For this review, take the finished solid that the model builds, in its own axes (mm). A direction names the side the tool comes from. Round coordinates to 2 decimals unless told otherwise and drop trailing zeros. Write each loop counter-clockwise with the first axis right and the second up, starting at its lowest first coordinate (ties: lowest second). Pieces come first, ordered by that corner, then holes. Notation, with made-up numbers: (43, 7.25) -> (102, 7.25) arc R34 ccw to (102, 46.25) -> close; hole circle Ø9 at (84, -10). An arc over 180 degrees is marked (long way). Write item = value, one per line. Start each with the question number.
```python
from build123d import *

# Parameters (mm, degrees)
SKETCH1_W           = 85.2
SKETCH1_H           = 85.2
BOSS_EXTRUDE1_DEPTH = 6.35
CUT_EXTRUDE1_REACH  = 62.579
SKETCH2_R           = 6.6675
CUT_EXTRUDE2_REACH  = 62.579
SKETCH3_R           = 2.6162
CUT_EXTRUDE3_REACH  = 62.579
SKETCH5_R           = 2.665
CIRPATTERN1_COUNT   = 4
CUT_EXTRUDE4_REACH  = 62.579
SKETCH6_W           = 85.2
SKETCH6_H           = 85.2
FILLET1_R           = 12.7


with BuildPart() as part:
    # Sketch1 → Boss-Extrude1 (new body)
    with BuildSketch(Plane(origin=(0, 0, 0), x_dir=(1, 0, 0), z_dir=(0, 1, 0))):
        Rectangle(SKETCH1_W, SKETCH1_H)
    extrude(amount=BOSS_EXTRUDE1_DEPTH)

    # Sketch2 → Cut-Extrude1 (cut, up to next)
    with BuildSketch(Plane(origin=(0, 6.35, 0), x_dir=(1, 0, 0), z_dir=(0, 1, 0)), mode=Mode.PRIVATE) as cut_extrude1_sk1:
        with Locations(Location((0, 0, 0), (0, 0, 270))):
            Circle(SKETCH2_R)
    cut_extrude1_tool1 = extrude(cut_extrude1_sk1.sketch, amount=-CUT_EXTRUDE1_REACH, mode=Mode.PRIVATE) & part.part
    add(cut_extrude1_tool1.solids().sort_by_distance((0, 6.35, 0))[0], mode=Mode.SUBTRACT)

    # Sketch3 → Cut-Extrude2 (cut, up to next)
    with BuildSketch(Plane(origin=(0, 6.35, 0), x_dir=(1, 0, 0), z_dir=(0, 1, 0)), mode=Mode.PRIVATE) as cut_extrude2_sk1:
        with Locations(Location((26.042742751, -26.042742751, 0), (0, 0, 270))):
            Circle(SKETCH3_R)
    cut_extrude2_tool1 = extrude(cut_extrude2_sk1.sketch, amount=-CUT_EXTRUDE2_REACH, mode=Mode.PRIVATE) & part.part
    # Sketch3 → Cut-Extrude2 (cut, up to next)
    with BuildSketch(Plane(origin=(0, 6.35, 0), x_dir=(1, 0, 0), z_dir=(0, 1, 0)), mode=Mode.PRIVATE) as cut_extrude2_sk2:
        with Locations(Location((-26.042742751, -26.042742751, 0), (0, 0, 270))):
            Circle(SKETCH3_R)
    cut_extrude2_tool2 = extrude(cut_extrude2_sk2.sketch, amount=-CUT_EXTRUDE2_REACH, mode=Mode.PRIVATE) & part.part
    # Sketch3 → Cut-Extrude2 (cut, up to next)
    with BuildSketch(Plane(origin=(0, 6.35, 0), x_dir=(1, 0, 0), z_dir=(0, 1, 0)), mode=Mode.PRIVATE) as cut_extrude2_sk3:
        with Locations(Location((26.042742751, 26.042742751, 0), (0, 0, 90))):
            Circle(SKETCH3_R)
    cut_extrude2_tool3 = extrude(cut_extrude2_sk3.sketch, amount=-CUT_EXTRUDE2_REACH, mode=Mode.PRIVATE) & part.part
    # Sketch3 → Cut-Extrude2 (cut, up to next)
    with BuildSketch(Plane(origin=(0, 6.35, 0), x_dir=(1, 0, 0), z_dir=(0, 1, 0)), mode=Mode.PRIVATE) as cut_extrude2_sk4:
        with Locations(Location((-26.042742751, 26.042742751, 0), (0, 0, 90))):
            Circle(SKETCH3_R)
    cut_extrude2_tool4 = extrude(cut_extrude2_sk4.sketch, amount=-CUT_EXTRUDE2_REACH, mode=Mode.PRIVATE) & part.part
    add(cut_extrude2_tool1.solids().sort_by_distance((26.042743, 6.35, 26.042743))[0], mode=Mode.SUBTRACT)
    add(cut_extrude2_tool2.solids().sort_by_distance((-26.042743, 6.35, 26.042743))[0], mode=Mode.SUBTRACT)
    add(cut_extrude2_tool3.solids().sort_by_distance((26.042743, 6.35, -26.042743))[0], mode=Mode.SUBTRACT)
    add(cut_extrude2_tool4.solids().sort_by_distance((-26.042743, 6.35, -26.042743))[0], mode=Mode.SUBTRACT)

    # Sketch5 → Cut-Extrude3 (cut, up to next)
    with BuildSketch(Plane(origin=(0, 6.35, 0), x_dir=(1, 0, 0), z_dir=(0, 1, 0)), mode=Mode.PRIVATE) as cut_extrude3_sk1:
        with Locations(Location((-34.75, -34.75, 0), (0, 0, 270))):
            Circle(SKETCH5_R)
    cut_extrude3_tool1 = extrude(cut_extrude3_sk1.sketch, amount=-CUT_EXTRUDE3_REACH, mode=Mode.PRIVATE) & part.part
    cut_extrude3 = cut_extrude3_tool1.solids().sort_by_distance((-34.75, 6.35, 34.75))[0]
    add(cut_extrude3, mode=Mode.SUBTRACT)

    # CirPattern1: Cut-Extrude3 ×4 about axis
    cirpattern1_axis = Axis((0, 0, 0), (0, 1, 0))
    for i in range(1, CIRPATTERN1_COUNT):
        add(cut_extrude3.rotate(cirpattern1_axis, i * 360 / CIRPATTERN1_COUNT), mode=Mode.SUBTRACT)

    # Sketch6 → Cut-Extrude4 (cut, up to next)
    with BuildSketch(Plane(origin=(0, 6.35, 0), x_dir=(1, 0, 0), z_dir=(0, 1, 0)), mode=Mode.PRIVATE) as cut_extrude4_sk1:
        Rectangle(SKETCH6_W, SKETCH6_H)
        with BuildLine():
            Line((31.75, -22.769743879), (39.240128061, -30.259871939))
            ThreePointArc((39.240128061, -30.259871939), (40.616635031, -32.319960204), (41.1, -34.75))
            ThreePointArc((41.1, -34.75), (37.180039796, -40.616635031), (30.259871939, -39.240128061))
            Line((30.259871939, -39.240128061), (22.769743879, -31.75))
            Line((22.769743879, -31.75), (-22.769743879, -31.75))
            Line((-22.769743879, -31.75), (-30.259871939, -39.240128061))
            ThreePointArc((-30.259871939, -39.240128061), (-39.240128061, -39.240128061), (-39.240128061, -30.259871939))
            Line((-39.240128061, -30.259871939), (-31.75, -22.769743879))
            Line((-31.75, -22.769743879), (-31.75, 22.769743879))
            Line((-31.75, 22.769743879), (-39.240128061, 30.259871939))
            ThreePointArc((-39.240128061, 30.259871939), (-39.240128061, 39.240128061), (-30.259871939, 39.240128061))
            Line((-30.259871939, 39.240128061), (-22.769743879, 31.75))
            Line((-22.769743879, 31.75), (22.769743879, 31.75))
            Line((22.769743879, 31.75), (30.259871939, 39.240128061))
            ThreePointArc((30.259871939, 39.240128061), (37.180039796, 40.616635031), (41.1, 34.75))
            ThreePointArc((41.1, 34.75), (40.616635031, 32.319960204), (39.240128061, 30.259871939))
            Line((39.240128061, 30.259871939), (31.75, 22.769743879))
            Line((31.75, 22.769743879), (31.75, -22.769743879))
        make_face(mode=Mode.SUBTRACT)
    cut_extrude4_tool1 = extrude(cut_extrude4_sk1.sketch, amount=-CUT_EXTRUDE4_REACH, mode=Mode.PRIVATE) & part.part
    add(cut_extrude4_tool1.solids().sort_by_distance((0, 6.35, 41.39509))[0], mode=Mode.SUBTRACT)

    # Fillet1
    fillet1_edges = [part.edges().sort_by_distance(p)[0] for p in [
        (22.769743879, 3.175, -31.75),
        (-22.769743879, 3.175, -31.75),
        (-31.75, 3.175, -22.769743879),
        (-31.75, 3.175, 22.769743879),
        (-22.769743879, 3.175, 31.75),
        (22.769743879, 3.175, 31.75),
        (31.75, 3.175, 22.769743879),
        (31.75, 3.175, -22.769743879),
    ]]
    fillet(fillet1_edges, radius=FILLET1_R)


solid = part.part
```
1. Clearance check with flat-ended pins moving along their axes: pin 1 Ø1.9 at (y, z) = (4, 8) entering from -X; pin 2 Ø3 at (y, z) = (4.5, -25.5) entering from -X; pin 3 Ø1.9 at (y, z) = (2, 2) entering from +X. State where each tip first meets the part, or that it passes through.
2. Consider section C-C, the plane z = -33.5. Give the boundary of the cut face in (x, y), then the cut area to 3 significant figures.
3. Consider section B-B, the plane z = 0. Give the boundary of the cut face in (x, y), then the cut area to 3 significant figures.
4. Machinability: for faces 5 (the flat face through (37.33, 3.22, 28.35)), 6 (the cylindrical face through (22.43, 3.13, 32.74)), 7 (the flat face through (-37.38, 3.22, 28.4)), 8 (the cylindrical face through (-39.14, 3.22, 39.34)), 9 (the flat face through (0, 3, -31.75)), which of the approach directions +Z, -Z, +X, -X, +Y, -Y give a long, thin tool a straight path to every point of the face, cutting with its end or side? Answer none if there is none.
5. Consider section D-D, the plane x = -27.5. Give the boundary of the cut face in (y, z), then the cut area to 3 significant figures.
6. Wall thickness on L1, parallel to X at y = 1.25, z = 11; L2, parallel to X at y = 6.25, z = 35; L3, parallel to Z at x = 5.5, y = 4: over which ranges is each line inside the solid? List them lowest first. Write a range as from..to.
7. Draft analysis for pull direction X (two halves, no side actions). For faces 1 (the cylindrical face through (22.3, 3.13, -32.69)), 2 (the cylindrical face through (-34.633, 3.219, 32.088)), 3 (the flat face through (-10, 0, -1)), 4 (the flat face through (-31.75, 3, 0)), state which applies: +X half, -X half, draft (parallel to the pull), parting line (faces both ways), or undercut.
8. Consider section A-A, the plane x = 0. Give the boundary of the cut face in (y, z), then the cut area to 3 significant figures.
Outcome:
q1.pin_1 = -31.75
q1.pin_2 = -35.98
q1.pin_3 = 31.75
q2.outline = (-40.98, 0) -> (-37.1, 0) -> (-37.1, 6.35) -> (-40.98, 6.35) -> close; (-32.4, 0) -> (-23.94, 0) -> (-23.94, 6.35) -> (-32.4, 6.35) -> close; (23.94, 0) -> (32.4, 0) -> (32.4, 6.35) -> (23.94, 6.35) -> close; (37.1, 0) -> (40.98, 0) -> (40.98, 6.35) -> (37.1, 6.35) -> close
q2.area = 157 mm2
q3.outline = (-31.75, 0) -> (-6.67, 0) -> (-6.67, 6.35) -> (-31.75, 6.35) -> close; (6.67, 0) -> (31.75, 0) -> (31.75, 6.35) -> (6.67, 6.35) -> close
q3.area = 319 mm2
q4.face_5 = +X, +Y, -Y
q4.face_6 = +Z, +Y, -Y
q4.face_7 = -X, +Y, -Y
q4.face_8 = +Y, -Y
q4.face_9 = -Z, +Y, -Y
q5.outline = (0, -36.48) -> (6.35, -36.48) -> (6.35, -28.22) -> (0, -28.22) -> close; (0, -23.87) -> (6.35, -23.87) -> (6.35, 23.87) -> (0, 23.87) -> close; (0, 28.22) -> (6.35, 28.22) -> (6.35, 36.48) -> (0, 36.48) -> close
q5.area = 408 mm2
q6.L1 = -31.75..31.75
q6.L2 = -41.1..-37.4, -32.1..-25.99, 25.99..32.1, 37.4..41.1
q6.L3 = -31.75..-3.77, 3.77..31.75
q7.face_1 = undercut
q7.face_2 = undercut
q7.face_3 = draft
q7.face_4 = -X half
q8.outline = (0, -31.75) -> (6.35, -31.75) -> (6.35, -6.67) -> (0, -6.67) -> close; (0, 6.67) -> (6.35, 6.67) -> (6.35, 31.75) -> (0, 31.75) -> close
q8.area = 319 mm2
